Read the model definition and answer for the solid it produces. Units are mm, in the model's axes. Face numbers are marked on the shaded views. A direction names the side the tool comes from. Round coordinates to 2 decimals unless told otherwise and drop trailing zeros. Order: outer loops, then holes, each group sorted by start corner. A loop starts at its lowest first (then second) coordinate and runs counter-clockwise, first axis right, second up. Notation, with made-up numbers: (77, 53) -> (93, 53) arc R24 ccw to (93, 89) -> close; hole circle Ø11 at (37, 48). An arc over 180 degrees is marked (long way). Use a Markdown table: item, result. Add a question column.
1. Consider L1, parallel to Y at x = 15, z = 5.25; L2, parallel to Y at x = -10, z = 3.25. Determine where each line is inside the solid, lowest interval first. Write a range as [from, to].
2. For the marked faces 1 and 2, determine the directions among +Z, -Z, +X, -X, +Y, -Y from which every point of the face is accessible in a straight line to the end or side of a thin tool.
3. Section B-B, the plane z = 5.5 is taken. Give the vertices of the cut face in (x, y).
4. Section A-A, the plane z = 1 is taken. Give the vertices of the cut face in (x, y), then the cut area to 3 significant figures.
5. The mould has two halves that part along Y. Classify the marked faces 3, 4 and 5: +Y half, -Y half, draft (parallel to the pull), parting line (faces both ways), or undercut.
6. Section C-C, the plane x = 2 is taken. Give the vertices of the cut face in (y, z), then the cut area to 3 significant figures.
7. Given pin 1 (21 mm diameter, centred on x = 7.5, y = 19, fed in from +Z); pin 2 (2 mm diameter, centred on y = -13.5, z = 1.5, fed in from -X); pin 3 (1 mm diameter, centred on y = 12, z = 1, fed in from +X), each flat-ended and moving along its own axis, determine where each tip first touches the part or whether it passes through.
8. Section D-D, the plane y = 24 is taken. Give the vertices of the cut face in (x, z).
```python
from build123d import *

# Parameters (mm, degrees)
SKETCH1_W           = 12.5
SKETCH1_H           = 30
SKETCH1_R           = 1.65
SKETCH1_W_2         = 30
SKETCH1_H_2         = 12.5
BOSS_EXTRUDE1_DEPTH = 6.5
SKETCH1_3_W         = 7.5
SKETCH1_3_H         = 30
SKETCH1_3_H_2       = 7.5
SKETCH1_3_W_2       = 30
BOSS_EXTRUDE2_DEPTH = 2
FILLET1_R           = 10
FILLET2_R           = 4
SKETCH2_R           = 3
CUT_EXTRUDE1_DEPTH  = 4.5
FILLET3_R           = 4
CUT_EXTRUDE2_DEPTH  = 2
FILLET4_R           = 2


with BuildPart() as part:
    # Sketch1 → Boss-Extrude1 (new body)
    # profile 1 of 3: a face of its own
    with BuildSketch(Plane.XY):
        with Locations((-13.75, 15)):
            Rectangle(SKETCH1_W, SKETCH1_H)
        with Locations(Location((-10, 15, 0), (0, 0, 180))):
            Circle(SKETCH1_R, mode=Mode.SUBTRACT)
    # profile 2 of 3: a face of its own
    with BuildSketch(Plane.XY):
        with BuildLine():
            Line((-7.5, 0), (-20, 0))
            Line((-20, 0), (-20, -10))
            ThreePointArc((-20, -10), (-17.071067812, -17.071067812), (-10, -20))
            Line((-10, -20), (0, -20))
            Line((0, -20), (0, -7.5))
            Line((0, -7.5), (-7.5, -7.5))
            Line((-7.5, -7.5), (-7.5, 0))
        make_face()
    # profile 3 of 3: a face of its own
    with BuildSketch(Plane.XY):
        with Locations((15, -13.75)):
            Rectangle(SKETCH1_W_2, SKETCH1_H_2)
        with Locations(Location((15, -10, 0), (0, 0, 180))):
            Circle(SKETCH1_R, mode=Mode.SUBTRACT)
    extrude(amount=BOSS_EXTRUDE1_DEPTH)

    # Sketch1<3> → Boss-Extrude2 (add)
    with BuildSketch(Plane.XY):
        with Locations((-3.75, 15)):
            Rectangle(SKETCH1_3_W, SKETCH1_3_H)
        with Locations((-3.75, -3.75)):
            Rectangle(SKETCH1_3_W, SKETCH1_3_H_2)
        with Locations((15, -3.75)):
            Rectangle(SKETCH1_3_W_2, SKETCH1_3_H_2)
        Polygon((0, 30), (30, 0), (0, 0), align=None)
    extrude(amount=BOSS_EXTRUDE2_DEPTH)

    # Fillet1
    fillet1_edges = [part.edges().sort_by_distance(p)[0] for p in [
        (30, 0, 1),
        (0, 30, 1),
    ]]
    fillet(fillet1_edges, radius=FILLET1_R)

    # Fillet2
    fillet2_edges = [part.edges().sort_by_distance(p)[0] for p in [
        (-20, 30, 3.25),
        (-7.5, 30, 4.25),
        (30, -7.5, 4.25),
        (30, -20, 3.25),
    ]]
    fillet(fillet2_edges, radius=FILLET2_R)

    # Sketch2 → Cut-Extrude1 (cut)
    with BuildSketch(Plane.XY.offset(6.5)):
        with Locations((-7.5, -7.5)):
            Circle(SKETCH2_R)
    extrude(amount=-CUT_EXTRUDE1_DEPTH, mode=Mode.SUBTRACT)

    # Fillet3
    fillet3_edges = [part.edges().sort_by_distance(p)[0] for p in [
        (-4.5, -7.5, 4.25),
        (-7.5, -4.5, 4.25),
    ]]
    fillet(fillet3_edges, radius=FILLET3_R)

    # Sketch3 → Cut-Extrude2 (cut)
    with BuildSketch(Plane.XY.offset(2)):
        Polygon((3.535533906, 0), (22.928932188, 0), (13.232233047, 9.696699141), align=None)
        Polygon((0, 22.928932188), (0, 3.535533906), (9.696699141, 13.232233047), align=None)
    extrude(amount=-CUT_EXTRUDE2_DEPTH, mode=Mode.SUBTRACT)

    # Fillet4
    fillet4_edges = [part.edges().sort_by_distance(p)[0] for p in [
        (0, 22.928932188, 1),
        (9.696699141, 13.232233047, 1),
        (0, 3.535533906, 1),
        (13.232233047, 9.696699141, 1),
        (22.928932188, 0, 1),
        (3.535533906, 0, 1),
    ]]
    fillet(fillet4_edges, radius=FILLET4_R)


solid = part.part
```
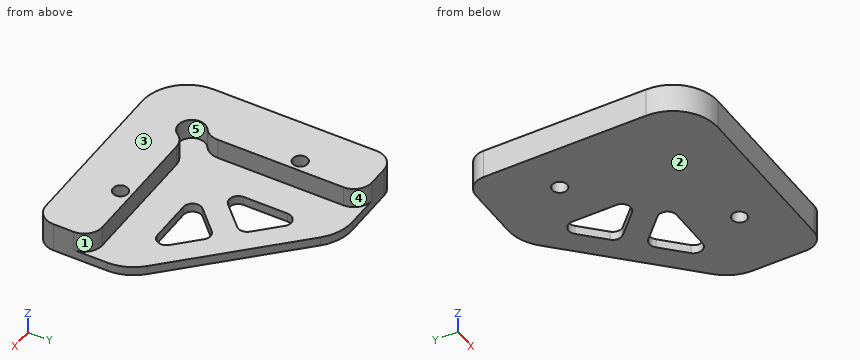
Verdict:
| question | item | result |
|---|---|---|
| 1 | L1 | y = [-20, -11.65], [-8.35, -7.5] |
| 1 | L2 | y = [-20, -9.16], [-5.84, 13.35], [16.65, 29.71] |
| 2 | face 1 | +Z, +X, +Y |
| 2 | face 2 | -Z, +X, -X, +Y, -Y |
| 3 | outline | (-20, -10) arc R10 ccw to (-10, -20) -> (26, -20) arc R4 ccw to (30, -16) -> (30, -11.5) arc R4 ccw to (26, -7.5) -> (-1.76, -7.5) arc R4 ccw to (-5.04, -9.21) arc R3 cw (long way) to (-9.21, -5.04) arc R4 ccw to (-7.5, -1.76) -> (-7.5, 26) arc R4 ccw to (-11.5, 30) -> (-16, 30) arc R4 ccw to (-20, 26) -> close; hole circle Ø3.3 at (-10, 15); hole circle Ø3.3 at (15, -10) |
| 4 | outline | (-20, -10) arc R10 ccw to (-10, -20) -> (26, -20) arc R4 ccw to (30, -16) -> (30, -4.14) arc R10 ccw to (27.07, 2.93) -> (2.93, 27.07) arc R10 ccw to (-4.14, 30) -> (-16, 30) arc R4 ccw to (-20, 26) -> close; hole circle Ø3.3 at (-10, 15); hole (0, 8.36) arc R2 ccw to (3.41, 6.95) -> (8.28, 11.82) arc R2 ccw to (8.28, 14.65) -> (3.41, 19.51) arc R2 ccw to (0, 18.1) -> close; hole (6.95, 3.41) arc R2 ccw to (8.36, 0) -> (18.1, 0) arc R2 ccw to (19.51, 3.41) -> (14.65, 8.28) arc R2 ccw to (11.82, 8.28) -> close; hole circle Ø3.3 at (15, -10) |
| 4 | area | 1,830 mm2 |
| 5 | face 3 | draft |
| 5 | face 4 | +Y half |
| 5 | face 5 | undercut |
| 6 | outline | (-20, 0) -> (6.36, 0) -> (6.36, 2) -> (-7.5, 2) -> (-7.5, 6.5) -> (-20, 6.5) -> close; (20.1, 0) -> (27.89, 0) -> (27.89, 2) -> (20.1, 2) -> close |
| 6 | area | 125 mm2 |
| 7 | pin 1 | stops at z = 2 |
| 7 | pin 2 | stops at x = -19.68 |
| 7 | pin 3 | stops at x = 18.5 |
| 8 | outline | (-20, 0) -> (6, 0) -> (6, 2) -> (-7.5, 2) -> (-7.5, 6.5) -> (-20, 6.5) -> close |
